Work out the finished part from the listing and answer in its coordinate system (mm). A direction names the side the tool comes from. Give positions to 0.01 mm unless a question says otherwise; leave off trailing zeros. Write each loop counter-clockwise with the first axis right and the second up, starting at its lowest first coordinate (ties: lowest second). Pieces come first, ordered by that corner, then holes.
1) Find section C-C (y = 4.25). Determine the outline of the cut face in (x, z) (3 decimals), plus the area to 3 significant figures.
2) Straight lines are drawn through the part: probe 1 along Y at (x, z) = (0, 4.75); probe 2 along Y at (x, z) = (-2.75, 6); probe 3 along Y at (x, z) = (4, 4.25). For each, find the intervals that lie inside material, in ascending order.
3) A tool of negligible diameter and unlimited length cuts with its end or side. For faces 1 (the face through (0.261, 6.345, 3.444)), 2 (the face through (1.27, -6, 4)), from which of +Z, -Z, +X, -X, +Y, -Y can it reach the whole face along a straight path? Write none if from no direction.
4) Find section A-A (x = 0). Count the separate pieces of the cut face and the enclosed holes in it, plus the area to 3 significant figures.
5) Given pin 1 Ø2 at (x, z) = (2.5, 1.5) entering from +Y; pin 2 Ø1 at (y, z) = (-3.5, 4) entering from -X; pin 3 Ø0.6 at (y, z) = (-5.5, 4) entering from +X, each flat-ended and moving along its own axis, determine where each tip first touches the part or whether it passes through.
```python
from build123d import *

# Parameters (mm, degrees)
F0_R     = 6.35
F1_DEPTH = 6.985
F2_R     = 0.9525
F3_DEPTH = 6.986
F5_DEPTH = 6.986


with BuildPart() as f1:
    # F0 (on Top) → F1 (new body)
    with BuildSketch(Plane.XY):
        Circle(F0_R)
    extrude(amount=F1_DEPTH)

    # F2 (on face) → F3 (cut, through all)
    with BuildSketch(Plane.XY.offset(6.985)):
        with Locations((0, 4.445)):
            Circle(F2_R)
        with Locations((3.14309, 3.14309)):
            Circle(F2_R)
        with Locations((3.14309, -3.14309)):
            Circle(F2_R)
        with Locations((-3.14309, 3.14309)):
            Circle(F2_R)
        with Locations((-3.14309, -3.14309)):
            Circle(F2_R)
        with Locations((-4.445, 0)):
            Circle(F2_R)
        with Locations((4.445, 0)):
            Circle(F2_R)
        Circle(F2_R)
    extrude(amount=-F3_DEPTH, mode=Mode.SUBTRACT)

    # F4 (on face) → F5 (cut, through all)
    with BuildSketch(Plane.XY.offset(6.985)):
        with BuildLine():
            Line((-1.27, -5.08), (-1.27, -6.221704))
            ThreePointArc((-1.27, -6.221704), (0, -6.35), (1.27, -6.221704))
            Line((1.27, -6.221704), (1.27, -5.08))
            Line((1.27, -5.08), (-1.27, -5.08))
        make_face()
    extrude(amount=-F5_DEPTH, mode=Mode.SUBTRACT)


solid = f1.part
```
Results:
1. outline: (-4.718, 0) - (-0.932, 0) - (-0.932, 6.985) - (-4.718, 6.985) - close; (0.932, 0) - (4.718, 0) - (4.718, 6.985) - (0.932, 6.985) - close
1. area: 52.9 mm2
2. probe 1: y = -5.08 to -0.95, 0.95 to 3.49, 5.4 to 6.35
2. probe 2: y = -5.72 to -4.01, -2.28 to 2.28, 4.01 to 5.72
2. probe 3: y = -4.93 to -3.56, -2.73 to -0.84, 0.84 to 2.73, 3.56 to 4.93
3. face 1: +Z, -Z
3. face 2: +Z, -Z, -Y
4. separate pieces: 3
4. enclosed holes: 0
4. area: 53.2 mm2
5. pin 1: stops at y = 6.17
5. pin 2: stops at x = -5.6
5. pin 3: stops at x = 3.64
